The drawing under review shows one solid part. Ordinate dimensions are in mm from its lowest x, y, z. A direction names the side the tool comes from. Coordinates: 2 decimals unless noted, no trailing zeros. Write each loop counter-clockwise with the first axis right and the second up, starting at its lowest first coordinate (ties: lowest second). Pieces come first, ordered by that corner, then holes.
1) For line 1 (X direction, y = 0.9, z = 13.5); line 2 (Y direction, x = 2.75, z = 4.5); line 3 (X direction, y = 2.75, z = 6.5), list the stretches that pass through material, from the lowest coordinate up.
2) Add section C-C, the plane y = 3.3. State the section outline as (x, z) points (1 decimal).
3) Add section D-D, the plane y = 5.1. State the section outline as (x, z) points.
4) Mouldability with a two-part tool opening along Z and no side actions: class the marked faces 1 and 2 as released by +Z, released by -Z, zero draft, split by the parting line, or undercut.
5) Add section A-A, the plane x = 2.75. State the section outline as (y, z) points.
6) Add section B-B, the plane z = 19. State the section outline as (x, y) points.
7) For P1, Ø2, axis at x = 2, y = 3.5, coming from the +Z side, flat-tipped, find the tip position at first contact; note if it passes through.
8) Machinability: for the marked faces 3, 4, 5, 6 and 7, which of the approach directions +Z, -Z, +X, -X, +Y, -Y give a long, thin tool a straight path to every point of the face, cutting with its end or side? Answer none if there is none.
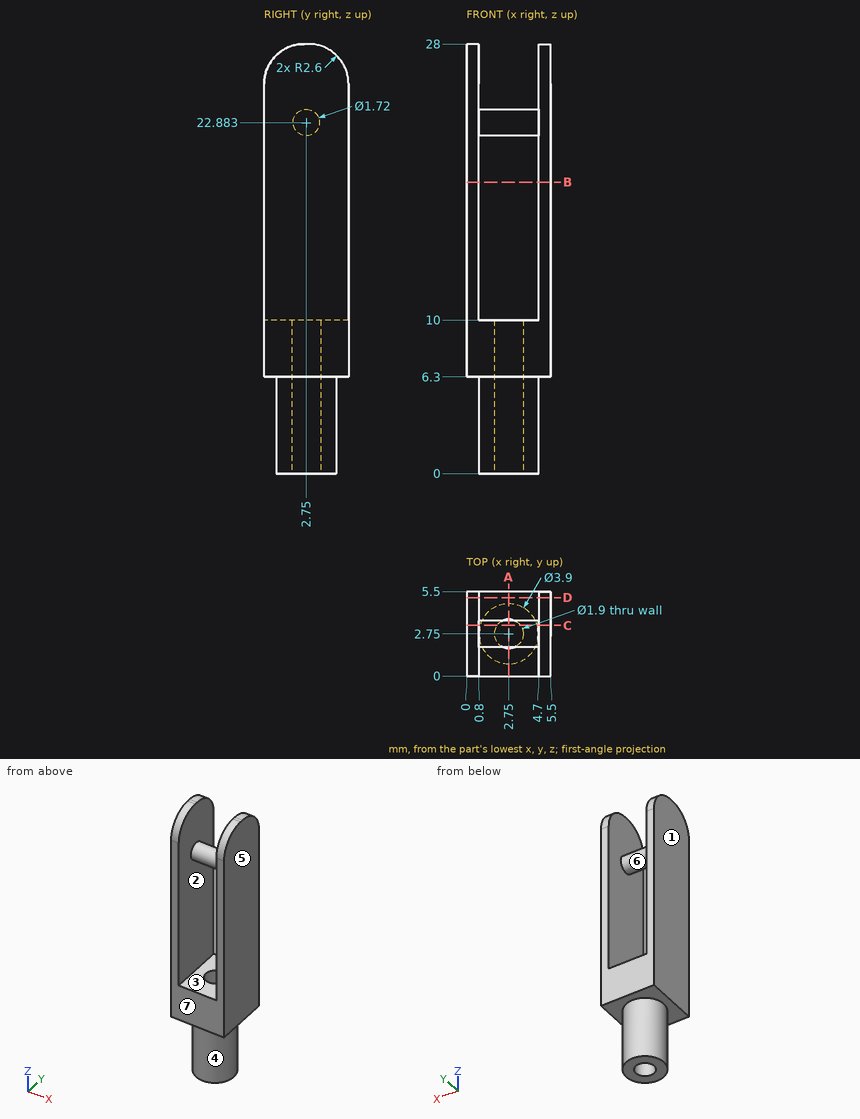
Geometry results:
1. line 1: x = 0 to 0.8, 4.7 to 5.5
1. line 2: y = 0.8 to 1.8, 3.7 to 4.7
1. line 3: x = 0 to 1.8, 3.7 to 5.5
2. outline: (0, 6.3) - (0.9, 6.3) - (0.9, 0) - (2, 0) - (2, 10) - (0.8, 10) - (0.8, 22.2) - (4.7, 22.2) - (4.7, 10) - (3.5, 10) - (3.5, 0) - (4.6, 0) - (4.6, 6.3) - (5.5, 6.3) - (5.5, 28) - (4.7, 28) - (4.7, 23.5) - (0.8, 23.5) - (0.8, 28) - (0, 28) - close
3. outline: (0, 6.3) - (5.5, 6.3) - (5.5, 26.79) - (4.7, 26.79) - (4.7, 10) - (0.8, 10) - (0.8, 26.79) - (0, 26.79) - close
4. face 1: zero draft
4. face 2: undercut
5. outline: (0, 6.3) - (0.8, 6.3) - (0.8, 0) - (1.8, 0) - (1.8, 10) - (0, 10) - close; circle Ø1.72 at (2.75, 22.88); (3.7, 0) - (4.7, 0) - (4.7, 6.3) - (5.5, 6.3) - (5.5, 10) - (3.7, 10) - close
6. outline: (0, 0) - (0.8, 0) - (0.8, 5.5) - (0, 5.5) - close; (4.7, 0) - (5.5, 0) - (5.5, 5.5) - (4.7, 5.5) - close
7. P1: stops at z = 23.74
8. face 3: +Y, -Y
8. face 4: -Z
8. face 5: +Z, -Z, +X, +Y, -Y
8. face 6: none
8. face 7: +Z, -Z, +X, -X, -Y
